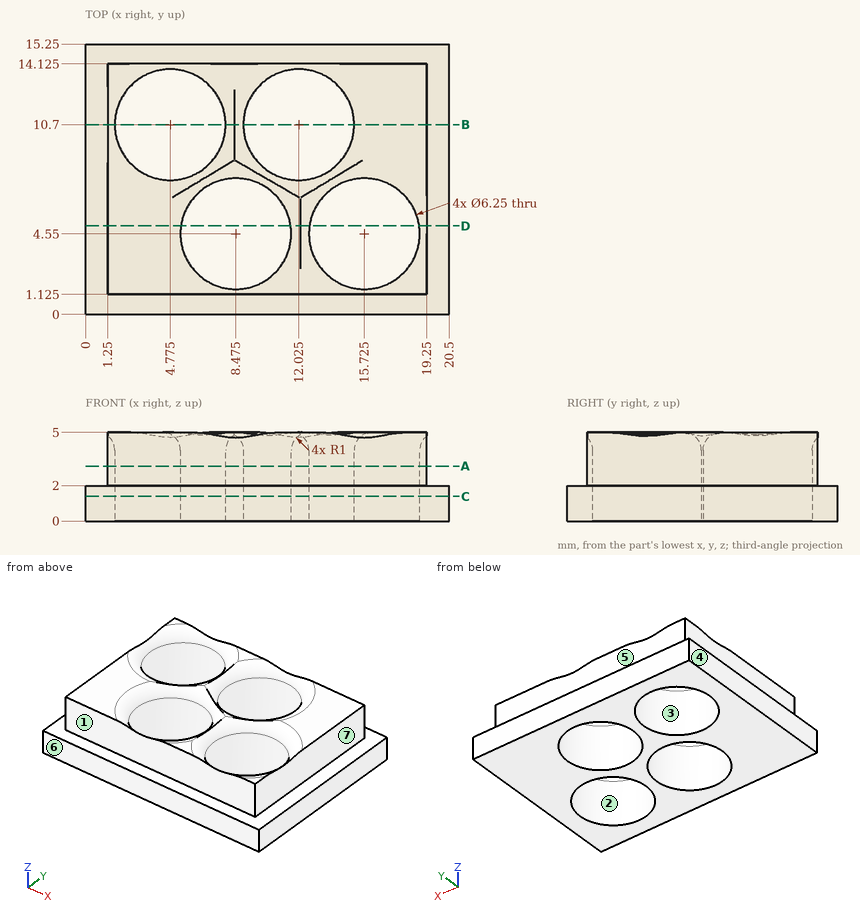
Print and shaded views of the part. All mm, measured from the part's lowest x, y and z. A direction names the side the tool comes from. Give positions to 0.01 mm unless a question says otherwise; leave off trailing zeros. Loops run counter-clockwise (first coordinate to the right, second up) from the corner with the lowest first, then second, coordinate; pieces in that order, holes last. Notation, with made-up numbers: (68, -6.75) - (78, -6.75) arc R10 cw to (78, 0.25) - close; hole circle Ø6 at (70, 10.5). An arc over 180 degrees is marked (long way). One line per item, written item: value. Start each with the question number.
1. Slice it at D-D (y = 5). Give the number of separate pieces and of enclosed holes in the cut face, plus the area to 3 significant figures.
2. Slice it at C-C (z = 1.4). List the corners of the cut face in (x, y) (3 decimals), plus the area to 3 significant figures.
3. Slice it at A-A (z = 3.1). List the corners of the cut face in (x, y) (3 decimals).
4. Pin check, flat tips, straight feed: pin 1 (3 mm diameter, centred on y = 9, z = 1.5, fed in from -X); pin 2 (1.5 mm diameter, centred on y = 7, z = 4, fed in from +X); pin 3 (1.5 mm diameter, centred on x = 14, z = 3, fed in from -Y) (3 decimals); pin 4 (5.5 mm diameter, centred on x = 4.775, y = 10.7, fed in from +Z). Stop position of each tip, or through.
5. Probe L1, parallel to X at y = 9.75, z = 0.6; L2, parallel to Y at x = 9.5, z = 1.1; L3, parallel to Y at x = 14.5, z = 3.6 (3 decimals). List the from-to ranges inside material, lowest first. Write a range as from..to.
6. Which spindle directions (+Z, -Z, +X, -X, +Y, -Y) get a long thin tool onto all of the face, cutting with end or side? Do the marked faces 5, 6 and 7. Say none if no direction does.
7. Pull direction X, two halves, no side cores. Call the marked faces 1, 2, 3 and 4: pulls with the +X half, pulls with the -X half, needs draft (parallel to the pull), parting line crosses it, or undercut.
8. Slice it at B-B (y = 10.7). List the corners of the cut face in (x, z).
Solution:
1. separate pieces: 3
1. enclosed holes: 0
1. area: 32.4 mm^2
2. outline: (0, 0) - (20.5, 0) - (20.5, 15.25) - (0, 15.25) - close; hole circle Ø6.25 at (4.775, 10.7); hole circle Ø6.25 at (8.475, 4.55); hole circle Ø6.25 at (12.025, 10.7); hole circle Ø6.25 at (15.725, 4.55)
2. area: 190 mm^2
3. outline: (1.25, 1.125) - (19.25, 1.125) - (19.25, 14.125) - (1.25, 14.125) - close; hole circle Ø6.25 at (4.775, 10.7); hole circle Ø6.25 at (8.475, 4.55); hole circle Ø6.25 at (12.025, 10.7); hole circle Ø6.25 at (15.725, 4.55)
4. pin 1: stops at x = 0
4. pin 2: stops at x = 19.25
4. pin 3: stops at y = 1.125
4. pin 4: passes through
5. L1: x = 0..1.8, 7.75..9.05, 15..20.5
5. L2: y = 0..1.6, 7.5..8.86, 12.54..15.25
5. L3: y = 1.125..1.675, 7.425..8.792, 12.608..14.125
6. face 5: +Z, +X, -X, +Y
6. face 6: +Z, -Z, +X, -X, -Y
6. face 7: +Z, +X, +Y, -Y
7. face 1: needs draft
7. face 2: undercut
7. face 3: undercut
7. face 4: pulls with the -X half
8. outline: (0, 0) - (1.65, 0) - (1.65, 4) arc R1 ccw to (1.25, 4.8) - (1.25, 2) - (0, 2) - close; (7.9, 0) - (8.9, 0) - (8.9, 4) arc R1 ccw to (8.4, 4.87) arc R1 ccw to (7.9, 4) - close; (15.15, 0) - (20.5, 0) - (20.5, 2) - (19.25, 2) - (19.25, 5) - (16.15, 5) arc R1 ccw to (15.15, 4) - close
